from build123d import *

# Parameters (mm, degrees)
F0_W     = 203.2
F0_H     = 101.6
F0_R     = 7.112
F1_DEPTH = 12.7
F2_W     = 12.7
F2_H     = 279.4
F3_DEPTH = 152.4
F4_SIZE  = 101.6
F5_SIZE  = 25.4


with BuildPart() as f1:
    # F0 (on Top) → F1 (new body)
    with BuildSketch(Plane.XY):
        Rectangle(F0_W, F0_H)
        with Locations((-76.2, -25.4)):
            Circle(F0_R, mode=Mode.SUBTRACT)
        with Locations((76.2, -25.4)):
            Circle(F0_R, mode=Mode.SUBTRACT)
        with Locations((-76.2, 25.4)):
            Circle(F0_R, mode=Mode.SUBTRACT)
        with Locations((76.2, 25.4)):
            Circle(F0_R, mode=Mode.SUBTRACT)
    extrude(amount=F1_DEPTH)

    # F2 (on face) → F3 (join)
    with BuildSketch(Plane(origin=(0, 0, 0), x_dir=(1, 0, 0), z_dir=(0, 0, -1))):
        with Locations((0, -88.9)):
            Rectangle(F2_W, F2_H)
    extrude(amount=F3_DEPTH)

    # F4
    f4_edges = [f1.edges().sort_by_distance(p)[0] for p in [
        (0, -50.8, -152.4),
    ]]
    chamfer(f4_edges, length=F4_SIZE)

    # F5
    f5_edges = [f1.edges().sort_by_distance(p)[0] for p in [
        (0, 228.6, 0),
    ]]
    chamfer(f5_edges, length=F5_SIZE)


solid = f1.part
Input: part model. Units: mm. Frame: model coordinates. A direction names the side the tool comes from. Round coordinates to 2 decimals unless told otherwise and drop trailing zeros. Loops run counter-clockwise (first coordinate to the right, second up) from the corner with the lowest first, then second, coordinate; pieces in that order, holes last. Notation, with made-up numbers: (19.25, 16.5) -> (68.25, 16.5) arc R17 cw to (68.25, 24.5) -> close; hole circle Ø6 at (76, 27). An arc over 180 degrees is marked (long way). Answer as a JSON object with one key per item and string values. Group by question number.
1) Ray query, L1, parallel to Y at x = -76.2, z = 4.5; L2, parallel to X at y = -25, z = 4; L3, parallel to Z at x = -57, y = -6. Return the intervals inside material, ascending.
2) Section query A-A on y = 25.4. Output: boundary loops of the cut face in (x, z).
3) Pin query (flat end, axial travel): pin 1 (6.5 mm diameter, centred on x = -2.5, y = 100, fed in from +Z); pin 2 (8 mm diameter, centred on y = 36.5, z = -124, fed in from -X); pin 3 (6.5 mm diameter, centred on x = -42.5, z = 5, fed in from +Y); pin 4 (13 mm diameter, centred on x = -76.2, y = -25.4, fed in from +Z). Return the tip coordinate at first contact, or that it passes through.
4) Reachability of faces 4 (the flat face through (0, 126, 0)), 5 (the flat face through (53, 1, 0)), 6 (the flat face through (-6.35, 91, -75)) from +Z, -Z, +X, -X, +Y, -Y: full face, straight path, thin tool, end or side. Return the list, or none.
5) Section query B-B on x = 76.2. Output: boundary loops of the cut face in (y, z).
6) Section query D-D on z = -134.5. Output: boundary loops of the cut face in (x, y).
7) Section query C-C on y = -25.4. Output: boundary loops of the cut face in (x, z).
8) Draft query along Y for faces 1 (the flat face through (6.35, 91, -75)), 2 (the cylindrical face through (82.984, 27.536, 6.261)), 3 (the flat face through (0, 228.6, -88)). Return one class per face: +Y half, -Y half, draft (parallel to the pull), parting line (faces both ways), or undercut.
Reply:
{
 "1": {"L1": "y = -50.8 to -32.51, -18.29 to 18.29, 32.51 to 50.8", "L2": "x = -101.6 to -83.3, -69.1 to 69.1, 83.3 to 101.6", "L3": "z = 0 to 12.7"},
 "2": {"outline": "(-101.6, 0) -> (-83.31, 0) -> (-83.31, 12.7) -> (-101.6, 12.7) -> close; (-69.09, 0) -> (-6.35, 0) -> (-6.35, -127) -> (6.35, -127) -> (6.35, 0) -> (69.09, 0) -> (69.09, 12.7) -> (-69.09, 12.7) -> close; (83.31, 0) -> (101.6, 0) -> (101.6, 12.7) -> (83.31, 12.7) -> close"},
 "3": {"pin 1": "stops at z = 0", "pin 2": "stops at x = -6.35", "pin 3": "stops at y = 50.8", "pin 4": "passes through"},
 "4": {"face 4": "+Z, +X, -X, +Y", "face 5": "-Z, +X, +Y, -Y", "face 6": "-Z, -X, +Y, -Y"},
 "5": {"outline": "(-50.8, 0) -> (-32.51, 0) -> (-32.51, 12.7) -> (-50.8, 12.7) -> close; (-18.29, 0) -> (18.29, 0) -> (18.29, 12.7) -> (-18.29, 12.7) -> close; (32.51, 0) -> (50.8, 0) -> (50.8, 12.7) -> (32.51, 12.7) -> close"},
 "6": {"outline": "(-6.35, 32.9) -> (6.35, 32.9) -> (6.35, 228.6) -> (-6.35, 228.6) -> close"},
 "7": {"outline": "(-101.6, 0) -> (-83.31, 0) -> (-83.31, 12.7) -> (-101.6, 12.7) -> close; (-69.09, 0) -> (-6.35, 0) -> (-6.35, -76.2) -> (6.35, -76.2) -> (6.35, 0) -> (69.09, 0) -> (69.09, 12.7) -> (-69.09, 12.7) -> close; (83.31, 0) -> (101.6, 0) -> (101.6, 12.7) -> (83.31, 12.7) -> close"},
 "8": {"face 1": "draft", "face 2": "undercut", "face 3": "+Y half"}
}
